The listing builds one solid part. Answer for the finished solid, in the listing's coordinates (mm). Face numbers are marked on the shaded views. A direction names the side the tool comes from. Coordinates: 2 decimals unless noted, no trailing zeros. Order: outer loops, then holes, each group sorted by start corner. A loop starts at its lowest first (then second) coordinate and runs counter-clockwise, first axis right, second up.
```python
from build123d import *

# Parameters (mm, degrees)
SKETCH1_R           = 1.450000001
SKETCH1_R_2         = 3.250000001
SKETCH1_R_3         = 1.5
SKETCH1_R_4         = 2.5
SKETCH1_R_5         = 1.375000001
BOSS_EXTRUDE2_DEPTH = 20


with BuildPart() as part:
    # Sketch1 → Boss-Extrude2 (new body)
    with BuildSketch(Plane.XY):
        with BuildLine():
            Line((-155.352886895, 10.211716756), (-51.913748531, 10.211716756))
            ThreePointArc((-51.913748531, 10.211716756), (-39.74822347, 6.086224622), (-32.601576204, -4.588283244))
            ThreePointArc((-32.601576204, -4.588283244), (53.610301025, -63.284580406), (124.587919611, 13.13479368))
            ThreePointArc((124.587919611, 13.13479368), (56.661218885, 95.304455124), (-32.601576204, 37.011716756))
            ThreePointArc((-32.601576204, 37.011716756), (-39.74822347, 26.33720889), (-51.913748531, 22.211716756))
            Line((-51.913748531, 22.211716756), (-155.352886895, 22.211716756))
            ThreePointArc((-155.352886895, 22.211716756), (-161.352886895, 16.211716756), (-155.352886895, 10.211716756))
        make_face()
        with Locations((-19.438766774, -20.788283242)):
            Circle(SKETCH1_R, mode=Mode.SUBTRACT)
        with Locations((-26.831398039, -2.940892579)):
            Circle(SKETCH1_R, mode=Mode.SUBTRACT)
        with Locations((-155.352886895, 16.211716756)):
            Circle(SKETCH1_R_2, mode=Mode.SUBTRACT)
        with Locations((-26.831398039, 35.364326096)):
            Circle(SKETCH1_R, mode=Mode.SUBTRACT)
        with Locations((-19.438766774, 53.211716759)):
            Circle(SKETCH1_R, mode=Mode.SUBTRACT)
        with Locations((-29.352886893, 16.211716758)):
            Circle(SKETCH1_R, mode=Mode.SUBTRACT)
        with Locations((44.647113106, 6.211716759)):
            Circle(SKETCH1_R_3, mode=Mode.SUBTRACT)
        with Locations((116.125624253, -2.940892579)):
            Circle(SKETCH1_R, mode=Mode.SUBTRACT)
        with Locations((108.732992988, -20.788283242)):
            Circle(SKETCH1_R, mode=Mode.SUBTRACT)
        with Locations((96.973014915, -36.114185049)):
            Circle(SKETCH1_R, mode=Mode.SUBTRACT)
        with Locations((81.647113106, -47.874163121)):
            Circle(SKETCH1_R, mode=Mode.SUBTRACT)
        with Locations((63.799722443, -55.266794386)):
            Circle(SKETCH1_R, mode=Mode.SUBTRACT)
        with Locations((44.647113106, -57.788283242)):
            Circle(SKETCH1_R, mode=Mode.SUBTRACT)
        with Locations((25.494503768, -55.266794386)):
            Circle(SKETCH1_R, mode=Mode.SUBTRACT)
        with Locations((7.647113108, -47.874163121)):
            Circle(SKETCH1_R, mode=Mode.SUBTRACT)
        with Locations((-7.678788702, -36.114185049)):
            Circle(SKETCH1_R, mode=Mode.SUBTRACT)
        with Locations((44.647113106, 16.211716756)):
            Circle(SKETCH1_R_4, mode=Mode.SUBTRACT)
        with Locations((-7.678788702, 68.537618566)):
            Circle(SKETCH1_R, mode=Mode.SUBTRACT)
        with Locations((7.647113108, 80.297596638)):
            Circle(SKETCH1_R, mode=Mode.SUBTRACT)
        with Locations((25.494503768, 87.690227903)):
            Circle(SKETCH1_R, mode=Mode.SUBTRACT)
        with Locations((44.647113106, 90.211716759)):
            Circle(SKETCH1_R, mode=Mode.SUBTRACT)
        with Locations((63.799722443, 87.690227903)):
            Circle(SKETCH1_R, mode=Mode.SUBTRACT)
        with Locations((81.647113106, 80.297596638)):
            Circle(SKETCH1_R, mode=Mode.SUBTRACT)
        with Locations((96.973014915, 68.537618566)):
            Circle(SKETCH1_R, mode=Mode.SUBTRACT)
        with Locations((108.732992988, 53.211716759)):
            Circle(SKETCH1_R, mode=Mode.SUBTRACT)
        with Locations((116.125624253, 35.364326096)):
            Circle(SKETCH1_R, mode=Mode.SUBTRACT)
        with Locations((44.647113106, 26.211716758)):
            Circle(SKETCH1_R_5, mode=Mode.SUBTRACT)
        with Locations((118.647113104, 16.211716758)):
            Circle(SKETCH1_R, mode=Mode.SUBTRACT)
        with BuildLine():
            Line((-4.014987137, 10.211716754), (22.197168785, 10.211716754))
            ThreePointArc((22.197168785, 10.211716754), (24.842920096, 9.454357441), (26.687157649, 7.411716754))
            ThreePointArc((26.687157649, 7.411716754), (44.647113107, -3.788283245), (62.607068564, 7.411716755))
            ThreePointArc((62.607068564, 7.411716755), (64.451306117, 9.454357442), (67.097057428, 10.211716755))
            Line((67.097057428, 10.211716755), (93.309213348, 10.211716755))
            ThreePointArc((93.309213348, 10.211716755), (105.842188723, 3.453350593), (107.081505871, -10.731679472))
            ThreePointArc((107.081505871, -10.731679472), (44.647113106, -51.788283245), (-17.787279658, -10.731679472))
            ThreePointArc((-17.787279658, -10.731679472), (-16.54796251, 3.453350591), (-4.014987137, 10.211716754))
        make_face(mode=Mode.SUBTRACT)
        with BuildLine():
            Line((93.309213348, 22.211716754), (67.097057429, 22.211716754))
            ThreePointArc((67.097057429, 22.211716754), (64.451306116, 22.969076068), (62.607068563, 25.011716756))
            ThreePointArc((62.607068563, 25.011716756), (44.647113106, 36.211716756), (26.68715765, 25.011716756))
            ThreePointArc((26.68715765, 25.011716756), (24.842920097, 22.969076069), (22.197168786, 22.211716756))
            Line((22.197168786, 22.211716756), (-4.014987136, 22.211716756))
            ThreePointArc((-4.014987136, 22.211716756), (-16.547962509, 28.970082919), (-17.787279657, 43.155112983))
            ThreePointArc((-17.787279657, 43.155112983), (44.647113107, 84.211716756), (107.08150587, 43.155112983))
            ThreePointArc((107.08150587, 43.155112983), (105.842188723, 28.970082917), (93.309213348, 22.211716754))
        make_face(mode=Mode.SUBTRACT)
    extrude(amount=BOSS_EXTRUDE2_DEPTH)


solid = part.part
```
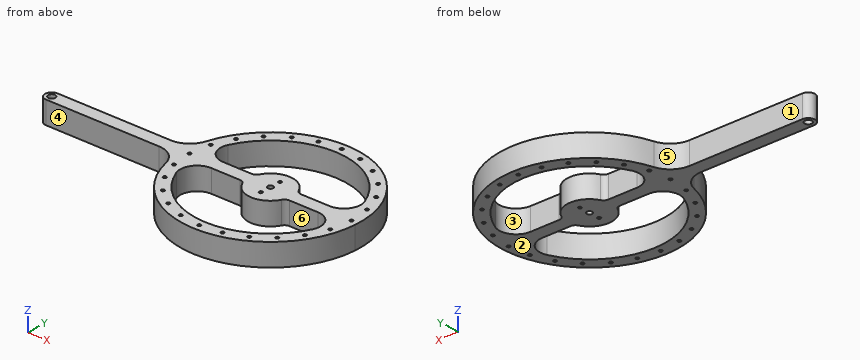
1) Straight lines are drawn through the part: probe 1 along Y at (x, z) = (94, 9.5); probe 2 along Y at (x, z) = (87.5, 14.25); probe 3 along X at (y, z) = (4.5, 13.5). For each, find the intervals that lie inside material, in ascending order.
2) A cutting plane is placed at D-D, the plane x = -98. Write down the section's boundary in (y, z).
3) A cutting plane is placed at A-A, the plane x = 31.5. Write down the section's boundary in (y, z).
4) A cutting plane is placed at B-B, the plane y = 75.5. Write down the section's boundary in (x, z).
5) For the marked faces 4, 5 and 6, determine the directions among +Z, -Z, +X, -X, +Y, -Y from which every point of the face is accessible in a straight line to the end or side of a thin tool.
6) The mould has two halves that part along Y. Classify the marked faces 1, 2 and 3: released by +Y, released by -Y, zero draft, split by the parting line, or undercut.
7) Each of these flat-tipped pins is pushed along its axis until it touches: P1, Ø2.5, axis at x = 44.65, y = 90.21, coming from the -Z side; P2, Ø3, axis at x = 44.65, y = 26.21, coming from the +Z side; P3, Ø2, axis at y = -17.5, z = 17, coming from the -X side; P4, Ø6, axis at x = -50.5, z = 5, coming from the -Y side. Where does it stop, or does it pass through?
8) A cutting plane is placed at C-C, the plane x = 75. Write down the section's boundary in (y, z), plus the area to 3 significant figures.
Working result:
1. probe 1: y = -46.75 to -30.57, 10.2 to 22.23, 62.99 to 79.17
1. probe 2: y = -51.34 to -36.59, 10.21 to 22.21, 69.01 to 83.77
1. probe 3: x = -37.92 to -15.79, 28.43 to 60.86, 105.09 to 123.79
2. outline: (10.21, 0) - (22.21, 0) - (22.21, 20) - (10.21, 20) - close
3. outline: (-62.7, 0) - (-50.51, 0) - (-50.51, 20) - (-62.7, 20) - close; (1.14, 0) - (31.28, 0) - (31.28, 20) - (1.14, 20) - close; (82.93, 0) - (95.12, 0) - (95.12, 20) - (82.93, 20) - close
4. outline: (-9.06, 0) - (11.35, 0) - (11.35, 20) - (-9.06, 20) - close; (77.95, 0) - (98.36, 0) - (98.36, 20) - (77.95, 20) - close
5. face 4: +Z, -Z, -X, -Y
5. face 5: +Z, -Z, -X, +Y
5. face 6: +Z, -Z
6. face 1: released by +Y
6. face 2: zero draft
6. face 3: undercut
7. P1: passes through
7. P2: stops at z = 20
7. P3: stops at x = -28.36
7. P4: stops at y = 9.72
8. outline: (-57.81, 0) - (-44.64, 0) - (-44.64, 20) - (-57.81, 20) - close; (10.21, 0) - (22.21, 0) - (22.21, 20) - (10.21, 20) - close; (77.06, 0) - (90.23, 0) - (90.23, 20) - (77.06, 20) - close
8. area: 767 mm2
